Here's how the part is built. I have some questions about the finished solid (model axes, mm). A direction names the side the tool comes from. Round coordinates to 2 decimals unless told otherwise and drop trailing zeros. Loops run counter-clockwise (first coordinate to the right, second up) from the corner with the lowest first, then second, coordinate; pieces in that order, holes last. Notation, with made-up numbers: M 58,-40 L 113,-40 A6 ccw 113,-33 Z; hole C 19.5,74 d6. An arc over 180 degrees is marked long. Use a Markdown table: item, result.
from build123d import *

# Parameters (mm, degrees)
SKETCH3_W                = 40
SKETCH3_H                = 30
SKETCH3_R                = 2.5
BOSS_EXTRUDE2_DEPTH      = 6.25
SKETCH4_W                = 40
SKETCH4_H                = 6.25
BOSS_EXTRUDE3_DEPTH      = 7.5
BOSS_EXTRUDE4_DEPTH      = 20
CHAMFER1_SIZE            = 2.5
SKETCH6_R                = 38
BOSS_EXTRUDE5_DEPTH      = 12.25
SKETCH8_R                = 28
BOSS_EXTRUDE7_DEPTH      = 10.5
SKETCH9_R                = 31.125
BOSS_EXTRUDE8_DEPTH      = 3.125
FILLET1_R                = 4
BOSS_EXTRUDE9_DEPTH      = 90
CHAMFER1_OF_MIRROR1_SIZE = 2.5
FILLET1_OF_MIRROR1_R     = 4
SKETCH12_R               = 2.5
BOSS_EXTRUDE10_DEPTH     = 30
SKETCH14_R               = 2.5
CUT_EXTRUDE1_DEPTH       = 10


with BuildPart() as part:
    # Sketch3 → Boss-Extrude2 (new body)
    with BuildSketch(Plane.XY):
        with Locations((0, -25)):
            Rectangle(SKETCH3_W, SKETCH3_H)
        with Locations((7.5, -25)):
            Circle(SKETCH3_R, mode=Mode.SUBTRACT)
        with Locations((-7.5, -25)):
            Circle(SKETCH3_R, mode=Mode.SUBTRACT)
    boss_extrude2 = extrude(amount=BOSS_EXTRUDE2_DEPTH)

    # Sketch4 → Boss-Extrude3 (add)
    with BuildSketch(Plane.XY.offset(6.25)):
        with Locations((0, -36.875)):
            Rectangle(SKETCH4_W, SKETCH4_H)
    boss_extrude3 = extrude(amount=BOSS_EXTRUDE3_DEPTH)

    # Sketch5 → Boss-Extrude4 (add)
    with BuildSketch(Plane.XY.offset(13.75)):
        Polygon((-20, -40), (-88.428700673, -40), (-107.5, -10), (-107.5, 10), (-110.625, 10), (-110.625, -10.909213368), (-90.145103003, -43.125), (90.145103003, -43.125), (110.625, -10.909213368), (110.625, 10), (107.5, 10), (107.5, -10), (88.428700673, -40), (20, -40), align=None)
    boss_extrude4 = extrude(amount=-BOSS_EXTRUDE4_DEPTH)

    # Chamfer1
    chamfer1_edges = [part.edges().sort_by_distance(p)[0] for p in [
        (-20, -40, 6.875),
        (-20, -10, 3.125),
        (20, -10, 3.125),
        (20, -40, 6.875),
    ]]
    chamfer(chamfer1_edges, length=CHAMFER1_SIZE)

    # Sketch6 → Boss-Extrude5 (add)
    with BuildSketch(Plane.XY.offset(13.75)):
        with BuildLine():
            Line((-110.625, 10), (-104.767593775, 21.060353399))
            ThreePointArc((-104.767593775, 21.060353399), (-50.991609061, 42.764061819), (-20.479289941, -6.550295858))
            ThreePointArc((-20.479289941, -6.550295858), (-19.779069285, -8.956923473), (-17.5, -10))
            Line((-17.5, -10), (17.5, -10))
            ThreePointArc((17.5, -10), (19.779069285, -8.956923473), (20.479289941, -6.550295858))
            ThreePointArc((20.479289941, -6.550295858), (50.991609061, 42.764061819), (104.767593775, 21.060353399))
            Line((104.767593775, 21.060353399), (110.625, 10))
            Line((110.625, 10), (110.625, -10.909213368))
            Line((110.625, -10.909213368), (90.145103003, -43.125))
            Line((90.145103003, -43.125), (-90.145103003, -43.125))
            Line((-90.145103003, -43.125), (-110.625, -10.909213368))
            Line((-110.625, -10.909213368), (-110.625, 10))
        make_face()
        with Locations((-65, 0)):
            Circle(SKETCH6_R, mode=Mode.SUBTRACT)
        with Locations(Location((65, 0, 0), (0, 0, 180))):
            Circle(SKETCH6_R, mode=Mode.SUBTRACT)
    boss_extrude5 = extrude(amount=BOSS_EXTRUDE5_DEPTH)

    # Sketch8 → Boss-Extrude7 (add)
    with BuildSketch(Plane.XY.offset(26)):
        with BuildLine():
            Line((-104.767593775, 21.060353399), (-110.625, 10))
            Line((-110.625, 10), (-110.625, -10.909213368))
            Line((-110.625, -10.909213368), (-90.145103003, -43.125))
            Line((-90.145103003, -43.125), (90.145103003, -43.125))
            Line((90.145103003, -43.125), (110.625, -10.909213368))
            Line((110.625, -10.909213368), (110.625, 10))
            Line((110.625, 10), (104.767593775, 21.060353399))
            ThreePointArc((104.767593775, 21.060353399), (50.991609061, 42.764061819), (20.479289941, -6.550295858))
            ThreePointArc((20.479289941, -6.550295858), (19.779069285, -8.956923473), (17.5, -10))
            Line((17.5, -10), (-17.5, -10))
            ThreePointArc((-17.5, -10), (-19.779069285, -8.956923473), (-20.479289941, -6.550295858))
            ThreePointArc((-20.479289941, -6.550295858), (-50.991609061, 42.764061819), (-104.767593775, 21.060353399))
        make_face()
        with Locations(Location((-65, 0, 0), (0, 0, 180))):
            Circle(SKETCH8_R, mode=Mode.SUBTRACT)
        with Locations(Location((65, 0, 0), (0, 0, 180))):
            Circle(SKETCH8_R, mode=Mode.SUBTRACT)
    boss_extrude7 = extrude(amount=BOSS_EXTRUDE7_DEPTH)

    # Sketch9 → Boss-Extrude8 (add)
    with BuildSketch(Plane.XY.offset(36.5)):
        with Locations(Location((65, 0, 0), (0, 0, 180))):
            Circle(SKETCH9_R)
        with Locations((-65, 0)):
            Circle(SKETCH9_R)
    boss_extrude8 = extrude(amount=BOSS_EXTRUDE8_DEPTH)

    # Fillet1
    # the kernel refuses this fillet: 4 mm, written as the material it adds along each edge
    with BuildSketch(Plane(origin=(-65, 0, 36.5), x_dir=(1, 0, 0), z_dir=(0, -1, 0))) as fillet1_piece_1:
        with BuildLine():
            CenterArc((35.028123749, 4), FILLET1_R, 192.635625093, 77.364374907)
            Line((31.125, 3.125), (31.046937525, 3.1075))
            ThreePointArc((31.046937525, 3.1075), (31.045, 1.5625), (31.045, 0))
            Line((31.045, 0), (31.125, -0.08))
            Line((31.125, -0.08), (35.028123749, -0.08))
            Line((35.028123749, -0.08), (35.028123749, 0))
        make_face()
    revolve(axis=Axis((-65, 0, 36.5), (0, 0, 1)))
    with BuildSketch(Plane(origin=(65, 0, 36.5), x_dir=(-1, 0, 0), z_dir=(0, 1, 0))) as fillet1_piece_2:
        with BuildLine():
            CenterArc((35.028123749, 4), FILLET1_R, 192.635625093, 77.364374907)
            Line((31.125, 3.125), (31.046937525, 3.1075))
            ThreePointArc((31.046937525, 3.1075), (31.045, 1.5625), (31.045, 0))
            Line((31.045, 0), (31.125, -0.08))
            Line((31.125, -0.08), (35.028123749, -0.08))
            Line((35.028123749, -0.08), (35.028123749, 0))
        make_face()
    revolve(axis=Axis((65, 0, 36.5), (0, 0, 1)))

    # Sketch10 → Boss-Extrude9 (add)
    with BuildSketch(Plane.XY.offset(36.5)):
        with BuildLine():
            Line((-104.767593775, 21.060353399), (-110.625, 10))
            Line((-110.625, 10), (-110.625, -10.909213368))
            Line((-110.625, -10.909213368), (-90.145103003, -43.125))
            Line((-90.145103003, -43.125), (-47.5, -43.125))
            Line((-47.5, -43.125), (-47.5, -40))
            Line((-47.5, -40), (-88.428700673, -40))
            Line((-88.428700673, -40), (-107.5, -10))
            Line((-107.5, -10), (-107.5, 9.223599474))
            Line((-107.5, 9.223599474), (-102.005955319, 19.597828858))
            ThreePointArc((-102.005955319, 19.597828858), (-51.964413987, 39.794335304), (-23.571005917, -6.095414201))
            ThreePointArc((-23.571005917, -6.095414201), (-22.144141184, -10.999485568), (-17.5, -13.125))
            Line((-17.5, -13.125), (17.5, -13.125))
            ThreePointArc((17.5, -13.125), (22.144141184, -10.999485568), (23.571005917, -6.095414201))
            ThreePointArc((23.571005917, -6.095414201), (51.964413987, 39.794335304), (102.005955319, 19.597828858))
            Line((102.005955319, 19.597828858), (107.5, 9.223599474))
            Line((107.5, 9.223599474), (107.5, -10))
            Line((107.5, -10), (88.428700673, -40))
            Line((88.428700673, -40), (47.5, -40))
            Line((47.5, -40), (47.5, -43.125))
            Line((47.5, -43.125), (90.145103003, -43.125))
            Line((90.145103003, -43.125), (110.625, -10.909213368))
            Line((110.625, -10.909213368), (110.625, 10))
            Line((110.625, 10), (104.767593775, 21.060353399))
            ThreePointArc((104.767593775, 21.060353399), (50.991609061, 42.764061819), (20.479289941, -6.550295858))
            ThreePointArc((20.479289941, -6.550295858), (19.779069285, -8.956923473), (17.5, -10))
            Line((17.5, -10), (-17.5, -10))
            ThreePointArc((-17.5, -10), (-19.779069285, -8.956923473), (-20.479289941, -6.550295858))
            ThreePointArc((-20.479289941, -6.550295858), (-50.991609061, 42.764061819), (-104.767593775, 21.060353399))
        make_face()
    boss_extrude9 = extrude(amount=BOSS_EXTRUDE9_DEPTH)

    # Mirror1: Boss-Extrude2, Boss-Extrude3, Boss-Extrude4, Boss-Extrude5, Boss-Extrude7, Boss-Extrude8, Boss-Extrude9 across plane
    add(boss_extrude2.mirror(Plane(origin=(-65, 0, 126.5), x_dir=(1, 0, 0), z_dir=(0, 0, 1))))
    add(boss_extrude3.mirror(Plane(origin=(-65, 0, 126.5), x_dir=(1, 0, 0), z_dir=(0, 0, 1))))
    add(boss_extrude4.mirror(Plane(origin=(-65, 0, 126.5), x_dir=(1, 0, 0), z_dir=(0, 0, 1))))
    add(boss_extrude5.mirror(Plane(origin=(-65, 0, 126.5), x_dir=(1, 0, 0), z_dir=(0, 0, 1))))
    add(boss_extrude7.mirror(Plane(origin=(-65, 0, 126.5), x_dir=(1, 0, 0), z_dir=(0, 0, 1))))
    add(boss_extrude8.mirror(Plane(origin=(-65, 0, 126.5), x_dir=(1, 0, 0), z_dir=(0, 0, 1))))
    add(boss_extrude9.mirror(Plane(origin=(-65, 0, 126.5), x_dir=(1, 0, 0), z_dir=(0, 0, 1))))

    # Chamfer1 of Mirror1
    chamfer1_of_mirror1_edges = [part.edges().sort_by_distance(p)[0] for p in [
        (-20, -40, 246.125),
        (-20, -10, 249.875),
        (20, -10, 249.875),
        (20, -40, 246.125),
    ]]
    chamfer(chamfer1_of_mirror1_edges, length=CHAMFER1_OF_MIRROR1_SIZE)

    # Fillet1 of Mirror1
    # the kernel refuses this fillet: 4 mm, written as the material it adds along each edge
    with BuildSketch(Plane(origin=(-65, 0, 216.5), x_dir=(1, 0, 0), z_dir=(0, -1, 0))) as fillet1_of_mirror1_piece_1:
        with BuildLine():
            CenterArc((35.028123749, -4), FILLET1_OF_MIRROR1_R, 90, 77.364374907)
            Line((31.125, -3.125), (31.046937525, -3.1075))
            ThreePointArc((31.046937525, -3.1075), (31.045, -1.5625), (31.045, 0))
            Line((31.045, 0), (31.125, 0.08))
            Line((31.125, 0.08), (35.028123749, 0.08))
            Line((35.028123749, 0.08), (35.028123749, 0))
        make_face()
    revolve(axis=Axis((-65, 0, 216.5), (0, 0, 1)))
    with BuildSketch(Plane(origin=(65, 0, 216.5), x_dir=(-1, 0, 0), z_dir=(0, 1, 0))) as fillet1_of_mirror1_piece_2:
        with BuildLine():
            CenterArc((35.028123749, -4), FILLET1_OF_MIRROR1_R, 90, 77.364374907)
            Line((31.125, -3.125), (31.046937525, -3.1075))
            ThreePointArc((31.046937525, -3.1075), (31.045, -1.5625), (31.045, 0))
            Line((31.045, 0), (31.125, 0.08))
            Line((31.125, 0.08), (35.028123749, 0.08))
            Line((35.028123749, 0.08), (35.028123749, 0))
        make_face()
    revolve(axis=Axis((65, 0, 216.5), (0, 0, 1)))

    # Sketch12 → Boss-Extrude10 (add)
    with BuildSketch(Plane.XY.offset(253)):
        Polygon((-20, -12.5), (-20, -37.5), (-22.5, -40), (22.5, -40), (20, -37.5), (20, -12.5), (17.5, -10), (-17.5, -10), align=None)
        with Locations((7.5, -25)):
            Circle(SKETCH12_R, mode=Mode.SUBTRACT)
        with Locations((-7.5, -25)):
            Circle(SKETCH12_R, mode=Mode.SUBTRACT)
    boss_extrude10 = extrude(amount=-BOSS_EXTRUDE10_DEPTH)

    # Mirror2: Boss-Extrude10 across plane
    add(boss_extrude10.mirror(Plane(origin=(0, 0, 126.5), x_dir=(1, 0, 0), z_dir=(0, 0, -1))))

    # Sketch14 → Cut-Extrude1 (cut)
    with BuildSketch(Plane.XZ.offset(43.125)):
        with Locations((10, 237.75)):
            Circle(SKETCH14_R)
        with Locations(Location((-10, 237.75, 0), (0, 0, 180))):
            Circle(SKETCH14_R)
        with Locations((-10, 15.25)):
            Circle(SKETCH14_R)
        with Locations(Location((10, 15.25, 0), (0, 0, 180))):
            Circle(SKETCH14_R)
    extrude(amount=-CUT_EXTRUDE1_DEPTH, mode=Mode.SUBTRACT)


solid = part.part
1. Imagine slicing it at B-B, the plane z = 64.5. Write out the boundary of the cut face in (x, y) (3 decimals).
Answer sheet:
| item | result |
|---|---|
| outline | M -110.625,-10.909 L -90.145,-43.125 L -47.5,-43.125 L -47.5,-40 L -88.429,-40 L -107.5,-10 L -107.5,9.224 L -102.006,19.598 A41.875 cw -23.571,-6.095 A6.136 ccw -17.5,-13.125 L 17.5,-13.125 A6.136 ccw 23.571,-6.095 A41.875 cw 102.006,19.598 L 107.5,9.224 L 107.5,-10 L 88.429,-40 L 47.5,-40 L 47.5,-43.125 L 90.145,-43.125 L 110.625,-10.909 L 110.625,10 L 104.768,21.06 A45 ccw 20.479,-6.55 A3.011 cw 17.5,-10 L -17.5,-10 A3.011 cw -20.479,-6.55 A45 ccw -104.768,21.06 L -110.625,10 Z |
2. For pin 1 Ø10 at (x, z) = (21, 253) entering from +Y; pin 2 Ø10 at (y, z) = (17.5, 121) entering from -X; pin 3 Ø4 at (x, y) = (-50, -31.5) entering from +Z, each with a flat end and sliding along its axis, tell me the tip position at first contact or that it passes through.
Answer sheet:
| item | result |
|---|---|
| pin 1 | y = -10 |
| pin 2 | x = -109.3 |
| pin 3 | z = 227 |
3. Which directions (+Z, -Z, +X, -X, +Y, -Y) give clear straight access to the entire face, cutting with the end or side of a thin tool? Please do faces 4 (the face through (-107.5, 0, 4)), 5 (the face through (-107.5, 0, 249)), 6 (the face through (65, 0, 39.625)).
Answer sheet:
| item | result |
|---|---|
| face 4 | -Z, +Y |
| face 5 | +Z, +Y |
| face 6 | none |
4. We'd pull the mould along X, two halves only. Please class faces 1 (the face through (-65, 0, 36.5)), 2 (the face through (107.74, 15.45, 128.08)), 3 (the face through (-1, -42, 259.25)): +X half, -X half, draft (parallel to the pull), parting line (faces both ways), or undercut.
Answer sheet:
| item | result |
|---|---|
| face 1 | undercut |
| face 2 | +X half |
| face 3 | draft |
5. Imagine slicing it at A-A, the plane y = 0. State how many separate pieces and enclosed holes the cut face has, then the cut area to 3 significant figures.
Answer sheet:
| item | result |
|---|---|
| separate pieces | 2 |
| enclosed holes | 2 |
| area | 5,470 mm2 |
6. I need wall thicknesses on probe 1 along Y at (x, z) = (65, 219.75) (3 decimals); probe 2 along X at (y, z) = (-25, 10.25); probe 3 along X at (y, z) = (19.5, 94). Which ranges of each line are inside material? Lowest first, please. Write a range as from..to.
Answer sheet:
| item | result |
|---|---|
| probe 1 | -43.125..-28, 28..45 |
| probe 2 | -101.67..-97.96, -20..-10, -5..5, 10..20, 97.96..101.67 |
| probe 3 | -105.59..-102.06, -27.94..-24.44, 24.44..27.94, 102.06..105.59 |
